Verification items for this drawing (mm, ordinates from the low corner). A direction names the side the tool comes from. Give positions to 0.01 mm unless a question says otherwise; leave off trailing zeros. Loops run counter-clockwise (first coordinate to the right, second up) from the corner with the lowest first, then second, coordinate; pieces in that order, holes last. Notation, with made-up numbers: (22.5, 19.25) -> (68.5, 19.25) arc R27 ccw to (68.5, 47.25) -> close; hole circle Ø7 at (87.5, -21.75). An arc over 180 degrees is marked (long way). Write item = value, one per line.
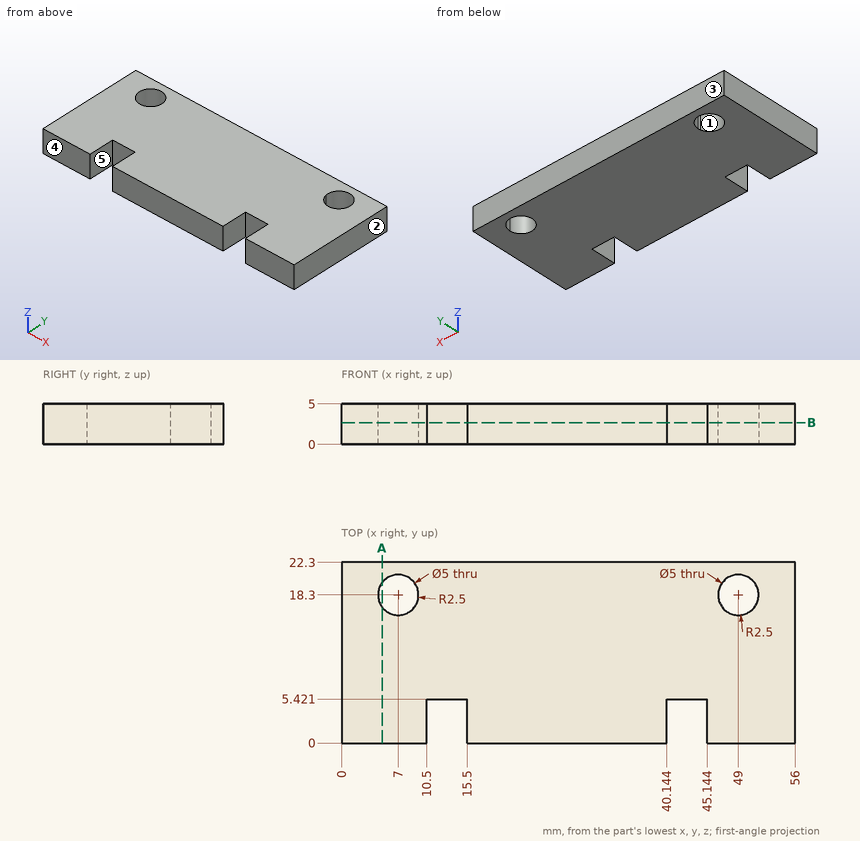
Item 1: Tool access check on the marked faces 4 and 5. Record the directions out of +Z, -Z, +X, -X, +Y, -Y that give a thin tool (end or side, any length) a straight path to the whole face; none if there is none.
Answer:
face_4 = +Z, -Z, +X, -X, -Y
face_5 = +Z, -Z, -Y
Item 2: Section check B-B, the plane z = 2.7. Record the cut outline in (x, y).
Answer:
outline = (0, 0) -> (10.5, 0) -> (10.5, 5.42) -> (15.5, 5.42) -> (15.5, 0) -> (40.14, 0) -> (40.14, 5.42) -> (45.14, 5.42) -> (45.14, 0) -> (56, 0) -> (56, 22.3) -> (0, 22.3) -> close; hole (9.44, 17.76) arc R2.5 ccw to (9.5, 18.3) arc R2.5 ccw (long way) to start; hole circle Ø5 at (49, 18.3)
Item 3: Draft check along X on the marked faces 1, 2 and 3. Enter one of: +X half, -X half, draft (parallel to the pull), parting line (faces both ways), or undercut.
Answer:
face_1 = undercut
face_2 = +X half
face_3 = draft
Item 4: Gauge pin test, flat ends, axial feed: pin 1 (1 mm diameter, centred on x = 8, z = 4, fed in from -Y); pin 2 (2.5 mm diameter, centred on x = 13, z = 2, fed in from -Y). Record the tip position at first contact, or that the pin passes through.
Answer:
pin_1 = 0
pin_2 = 5.42
Item 5: Thickness scan on L1, parallel to X at y = 18.3, z = 1.85; L2, parallel to X at y = 1.5, z = 4.6; L3, parallel to Y at x = 49, z = 3.4. Record the ranges inside material, lowest first. Write a range as [from, to].
Answer:
L1 = [0, 4.5], [9.5, 46.5], [51.5, 56]
L2 = [0, 10.5], [15.5, 40.14], [45.14, 56]
L3 = [0, 15.8], [20.8, 22.3]
Item 6: Section check A-A, the plane x = 5. Record the cut outline in (y, z).
Answer:
outline = (0, 0) -> (16.8, 0) -> (16.8, 5) -> (0, 5) -> close; (19.8, 0) -> (22.3, 0) -> (22.3, 5) -> (19.8, 5) -> close
